```python
from build123d import *

# Parameters (mm, degrees)
SKETCH1_R           = 7.5
BOSS_EXTRUDE1_DEPTH = 10
CHAMFER1_SIZE       = 2


with BuildPart() as part:
    # Sketch1 → Boss-Extrude1 (new body)
    with BuildSketch(Plane.XY):
        Polygon((7.216878365, -12.5), (14.43375673, 0), (7.216878365, 12.5), (-7.216878365, 12.5), (-14.43375673, 0), (-7.216878365, -12.5), align=None)
        Circle(SKETCH1_R, mode=Mode.SUBTRACT)
    extrude(amount=BOSS_EXTRUDE1_DEPTH)

    # Chamfer1
    chamfer1_edges = [part.edges().sort_by_distance(p)[0] for p in [
        (10.825317547, 6.25, 10),
        (0, 12.5, 10),
        (-10.825317547, 6.25, 10),
        (-10.825317547, -6.25, 10),
        (0, -12.5, 10),
        (10.825317547, -6.25, 10),
    ]]
    chamfer(chamfer1_edges, length=CHAMFER1_SIZE)


solid = part.part
```
Work out the finished part from the listing and answer in its coordinate system (mm). Give positions to 0.01 mm unless a question says otherwise; leave off trailing zeros. Loops run counter-clockwise (first coordinate to the right, second up) from the corner with the lowest first, then second, coordinate; pieces in that order, holes last. Notation, with made-up numbers: (31, 36) -> (61, 36) arc R15 ccw to (61, 46) -> close; hole circle Ø7 at (10.5, -26). An arc over 180 degrees is marked (long way). Use CSV: the item, a comma, the result in double quotes.
1. The part is cut by section D-D (z = 9.25). Write down the section's boundary in (x, y).
Found:
outline,"(-12.99, 0) -> (-6.5, -11.25) -> (6.5, -11.25) -> (12.99, 0) -> (6.5, 11.25) -> (-6.5, 11.25) -> close; hole circle Ø15 at (0, 0)"
2. The part is cut by section C-C (z = 3.25). Write down the section's boundary in (x, y).
Found:
outline,"(-14.43, 0) -> (-7.22, -12.5) -> (7.22, -12.5) -> (14.43, 0) -> (7.22, 12.5) -> (-7.22, 12.5) -> close; hole circle Ø15 at (0, 0)"
3. The mould has two halves that part along X. Classify faces 1 (the flat face through (10, 5.66, 9.01)), 2 (the cylindrical face through (-7.493, 0.33, 4.93)), 3 (the flat face through (-0.1, -11.5, 9)): +X half, -X half, draft (parallel to the pull), parting line (faces both ways), or undercut.
Found:
face 1,"+X half"
face 2,"undercut"
face 3,"draft"
4. The part is cut by section B-B (y = -5.5). Write down the section's boundary in (x, z), then the cut area to 3 significant figures.
Found:
outline,"(-11.26, 0) -> (-5.1, 0) -> (-5.1, 10) -> (-8.95, 10) -> (-11.26, 8) -> close; (5.1, 0) -> (11.26, 0) -> (11.26, 8) -> (8.95, 10) -> (5.1, 10) -> close"
area,"119 mm^2"
5. The part is cut by section A-A (x = 0). Write down the section's boundary in (y, z).
Found:
outline,"(-12.5, 0) -> (-7.5, 0) -> (-7.5, 10) -> (-10.5, 10) -> (-12.5, 8) -> close; (7.5, 0) -> (12.5, 0) -> (12.5, 8) -> (10.5, 10) -> (7.5, 10) -> close"
6. Flat-ended cylindrical pins translate along their axes: pin 1 Ø6 at (y, z) = (9, 4.5) entering from +X; pin 2 Ø2 at (x, z) = (-10, 7) entering from +Y; pin 3 Ø2 at (x, z) = (-9.5, 5.5) entering from -Y. Find the tip coordinate at first contact, or state that the pin passes through.
Found:
pin 1,"x = 10.97"
pin 2,"y = 9.41"
pin 3,"y = -10.28"
7. Straight lines are drawn through the part: line 1 (Y direction, x = 0, z = 6.25); line 2 (X direction, y = 0.75, z = 9.25); line 3 (X direction, y = 1.5, z = 7.5). For each, find the intervals that lie inside material, in ascending order.
Found:
line 1,"-12.5 to -7.5, 7.5 to 12.5"
line 2,"-12.56 to -7.46, 7.46 to 12.56"
line 3,"-13.57 to -7.35, 7.35 to 13.57"
